from build123d import *

# Parameters (mm, degrees)
SKETCH1_W               = 101.6
SKETCH1_H               = 50.8
BOSS_EXTRUDE1_DEPTH     = 0.3175
SKETCH2_R               = 2.032
CUT_EXTRUDE1_DEPTH      = 57.799676275
MIRROR2_COPY_1_SKETCH_R = 2.032
MIRROR2_COPY_1_DEPTH    = 57.799676275
SKETCH3_W               = 86.868
SKETCH3_H               = 43.688
BOSS_EXTRUDE2_DEPTH     = 2.54
SKETCH3_2_W             = 86.868
SKETCH3_2_H             = 43.688
BOSS_EXTRUDE3_DEPTH     = 30.226
FILLET1_R               = 2.54


with BuildPart() as part:
    # Sketch1 → Boss-Extrude1 (new, symmetric)
    with BuildSketch(Plane(origin=(0, 0, 0), x_dir=(1, 0, 0), z_dir=(0, 1, 0))):
        Rectangle(SKETCH1_W, SKETCH1_H)
    extrude(amount=BOSS_EXTRUDE1_DEPTH, both=True)

    # Sketch2 → Cut-Extrude1 (cut, through all)
    with BuildSketch(Plane(origin=(0, 0.3175, 0), x_dir=(1, 0, 0), z_dir=(0, 1, 0))):
        with Locations(Location((-47.244, -21.844, 0), (0, 0, 270))):
            Circle(SKETCH2_R)
    cut_extrude1 = extrude(amount=-CUT_EXTRUDE1_DEPTH, mode=Mode.SUBTRACT)

    # Mirror1: Cut-Extrude1 across plane
    add(cut_extrude1.mirror(Plane.XY), mode=Mode.SUBTRACT)

    # Mirror2: Cut-Extrude1 across plane
    add(cut_extrude1.mirror(Plane(origin=(0, 0, 0), x_dir=(0, 0, 1), z_dir=(1, 0, 0))), mode=Mode.SUBTRACT)

    # Mirror2 copy 1 sketch → Mirror2 copy 1 (cut, through all)
    with BuildSketch(Plane(origin=(0, 0.3175, 0), x_dir=(-1, 0, 0), z_dir=(0, 1, 0))):
        with Locations(Location((-47.244, -21.844, 0), (0, 0, 270))):
            Circle(MIRROR2_COPY_1_SKETCH_R)
    extrude(amount=-MIRROR2_COPY_1_DEPTH, mode=Mode.SUBTRACT)

    # Sketch3 → Boss-Extrude2 (add)
    with BuildSketch(Plane(origin=(0, 0, 0), x_dir=(1, 0, 0), z_dir=(0, 1, 0))):
        Rectangle(SKETCH3_W, SKETCH3_H)
    extrude(amount=-BOSS_EXTRUDE2_DEPTH)

    # Sketch3<2> → Boss-Extrude3 (add)
    with BuildSketch(Plane(origin=(0, 0, 0), x_dir=(1, 0, 0), z_dir=(0, 1, 0))):
        Rectangle(SKETCH3_2_W, SKETCH3_2_H)
    extrude(amount=BOSS_EXTRUDE3_DEPTH)

    # Fillet1
    fillet1_edges = [part.edges().sort_by_distance(p)[0] for p in [
        (43.434, 15.27175, 21.844),
        (43.434, 15.27175, -21.844),
        (-43.434, 15.27175, -21.844),
        (-43.434, 15.27175, 21.844),
        (43.434, 30.226, 0),
        (0, 30.226, -21.844),
        (-43.434, 30.226, 0),
        (0, 30.226, 21.844),
    ]]
    fillet(fillet1_edges, radius=FILLET1_R)


solid = part.part
Read the model definition and answer for the solid it produces. Units are mm, in the model's axes. A direction names the side the tool comes from. Round coordinates to 2 decimals unless told otherwise and drop trailing zeros. Order: outer loops, then holes, each group sorted by start corner. A loop starts at its lowest first (then second) coordinate and runs counter-clockwise, first axis right, second up.
1) Straight lines are drawn through the part: L1, parallel to Z at x = 29, y = 27.5; L2, parallel to X at y = -0.5, z = -0.5; L3, parallel to Y at x = -2, z = -19.5. For each, find the intervals that lie inside material, in ascending order.
2) The part is cut by section C-C on y = 25. Write down the section's boundary in (x, z).
3) The part is cut by section A-A on x = -14. Write down the section's boundary in (y, z), plus the area to 3 significant figures.
4) For faces 5 (the face through (-1, 14, -21.844)), 6 (the face through (-42.71, 14.19, -21.08)), 7 (the face through (42.67, 14.19, 21.12)), 8 (the face through (43.434, -1, 0)), 9 (the face through (-1, 0.318, 22)), determine the directions among +Z, -Z, +X, -X, +Y, -Y from which every point of the face is accessible in a straight line to the end or side of a thin tool.
5) The mould has two halves that part along Z. Classify faces 1 (the face through (-1, -1, -21.844)), 2 (the face through (-1, 30.226, 0)), 3 (the face through (-1, 14, 21.844)), 4 (the face through (45.23, 0, -21.58)): released by +Z, released by -Z, zero draft, split by the parting line, or undercut.
6) Flat-ended cylindrical pins translate along their axes: pin 1 (2.5 mm diameter, centred on y = -1.5, z = 7.5, fed in from +X); pin 2 (13.5 mm diameter, centred on x = 4.5, y = 8, fed in from +Z); pin 3 (6 mm diameter, centred on y = 26.5, z = 15, fed in from -X); pin 4 (2.5 mm diameter, centred on x = -47.244, z = 21.844, fed in from +Y). Find the tip coordinate at first contact, or state that the pin passes through.
7) The part is cut by section B-B on z = -17.5. Write down the section's boundary in (x, y), plus the area to 3 significant figures.
Resolved:
1. L1: z = -21.84 to 21.84
1. L2: x = -43.43 to 43.43
1. L3: y = -2.54 to 30.22
2. outline: (-43.43, -19.3) arc R2.54 ccw to (-40.89, -21.84) - (40.89, -21.84) arc R2.54 ccw to (43.43, -19.3) - (43.43, 19.3) arc R2.54 ccw to (40.89, 21.84) - (-40.89, 21.84) arc R2.54 ccw to (-43.43, 19.3) - close
3. outline: (-2.54, -21.84) - (-0.32, -21.84) - (-0.32, -25.4) - (0.32, -25.4) - (0.32, -21.84) - (27.69, -21.84) arc R2.54 ccw to (30.23, -19.3) - (30.23, 19.3) arc R2.54 ccw to (27.69, 21.84) - (0.32, 21.84) - (0.32, 25.4) - (-0.32, 25.4) - (-0.32, 21.84) - (-2.54, 21.84) - close
3. area: 1,430 mm2
4. face 5: -Z, +X, -X, +Y
4. face 6: -Z, -X, +Y
4. face 7: +Z, +X, +Y
4. face 8: +Z, -Z, +X, -Y
4. face 9: +Y
5. face 1: released by -Z
5. face 2: zero draft
5. face 3: released by +Z
5. face 4: undercut
6. pin 1: stops at x = 50.8
6. pin 2: stops at z = 21.84
6. pin 3: stops at x = -43.43
6. pin 4: passes through
7. outline: (-50.8, -0.32) - (-43.43, -0.32) - (-43.43, -2.54) - (43.43, -2.54) - (43.43, -0.32) - (50.8, -0.32) - (50.8, 0.32) - (43.43, 0.32) - (43.43, 27.69) arc R2.54 ccw to (40.89, 30.23) - (-40.89, 30.23) arc R2.54 ccw to (-43.43, 27.69) - (-43.43, 0.32) - (-50.8, 0.32) - close
7. area: 2,850 mm2
